from build123d import *

# Parameters (mm, degrees)
Y_KSEKLIK_EKSTR_ZYON1_DEPTH = 2.5
IZIM2_R                     = 1.5
KES_EKSTR_ZYON1_DEPTH       = 11
IZIM3_W                     = 10
IZIM3_H                     = 15
Y_KSEKLIK_EKSTR_ZYON2_DEPTH = 15
IZIM4_W                     = 10
IZIM4_H                     = 10
KES_EKSTR_ZYON2_DEPTH       = 10
IZIM5_R                     = 1.5
KES_EKSTR_ZYON3_DEPTH       = 18


with BuildPart() as part:
    # Çizim1 → Yükseklik-Ekstrüzyon1 (new, symmetric)
    with BuildSketch(Plane.XY):
        with BuildLine():
            Line((22.660097643, 2.30045544), (29.392284146, 8.057892583))
            ThreePointArc((29.392284146, 8.057892583), (30.202384575, 13.188927169), (25.261772713, 14.793337669))
            Line((25.261772713, 14.793337669), (0, 4.329568801))
            Line((0, 4.329568801), (-25.261772713, 14.793337669))
            ThreePointArc((-25.261772713, 14.793337669), (-30.21464291, 13.168805295), (-29.356291498, 8.02747653))
            ThreePointArc((-29.356291498, 8.02747653), (-15.084034375, -6.132217103), (-5, -23.524931034))
            Line((-5, -23.524931034), (-5, -63.524931034))
            Line((-5, -63.524931034), (5, -63.524931034))
            Line((5, -63.524931034), (5, -23.524931034))
            ThreePointArc((5, -23.524931034), (12.493835858, -9.698499239), (22.660097643, 2.30045544))
        make_face()
    extrude(amount=Y_KSEKLIK_EKSTR_ZYON1_DEPTH, both=True)

    # Çizim2 → Kes-Ekstrüzyon1 (cut, symmetric)
    with BuildSketch(Plane.XY.offset(2.5)):
        with Locations((-26.792506443, 11.097819539)):
            Circle(IZIM2_R)
        with Locations((26.792506443, 11.097819539)):
            Circle(IZIM2_R)
    extrude(amount=KES_EKSTR_ZYON1_DEPTH, both=True, mode=Mode.SUBTRACT)

    # Çizim3 → Yükseklik-Ekstrüzyon2 (add)
    with BuildSketch(Plane.XZ.offset(63.524931034)):
        Rectangle(IZIM3_W, IZIM3_H)
    extrude(amount=Y_KSEKLIK_EKSTR_ZYON2_DEPTH)

    # Çizim4 → Kes-Ekstrüzyon2 (cut)
    with BuildSketch(Plane.XZ.offset(78.524931034)):
        Rectangle(IZIM4_W, IZIM4_H)
    extrude(amount=-KES_EKSTR_ZYON2_DEPTH, mode=Mode.SUBTRACT)

    # Çizim5 → Kes-Ekstrüzyon3 (cut)
    with BuildSketch(Plane.XY.offset(7.5)):
        with Locations((0, -73.524931034)):
            Circle(IZIM5_R)
    extrude(amount=-KES_EKSTR_ZYON3_DEPTH, mode=Mode.SUBTRACT)


solid = part.part
Verification items for the finished model (mm, model axes). A direction names the side the tool comes from. Coordinates: 2 decimals unless noted, no trailing zeros. Write each loop counter-clockwise with the first axis right and the second up, starting at its lowest first coordinate (ties: lowest second). Pieces come first, ordered by that corner, then holes. Notation, with made-up numbers: M 26,66.25 L 31,66.25 A29 cw 31,95.25 Z; hole C -35,44.5 d10. An arc over 180 degrees is marked long. Use a Markdown table: item, result.
Q1. Set-up check for faces 1 (the face through (-5, -55, 0)), 2 (the face through (0, -12, -2.5)), 3 (the face through (0, -12, 2.5)), 4 (the face through (12.808, 9.635, 0.035)), 5 (the face through (-1, -75, -5)): record each of +Z, -Z, +X, -X, +Y, -Y from which the full face is reachable in a straight line by a thin tool's end or side.
Reply:
| item | result |
|---|---|
| face 1 | +Z, -Z, -X, -Y |
| face 2 | -Z, +X, -X, +Y |
| face 3 | +Z, +X, -X, +Y |
| face 4 | +Z, -Z, +Y |
| face 5 | +X, -X, -Y |
Q2. Thickness scan on line 1 (Y direction, x = 0, z = -6.2); line 2 (Z direction, x = 1, y = -54.5); line 3 (X direction, y = -58.5, z = 2). Record the ranges inside material, lowest first.
Reply:
| item | result |
|---|---|
| line 1 | y = -78.52 to -75.02, -72.02 to -63.52 |
| line 2 | z = -2.5 to 2.5 |
| line 3 | x = -5 to 5 |
Q3. Go/stop test with flat-tipped pins: P1, Ø5, axis at x = -0.5, y = -72.5, coming from the +Z side; P2, Ø5, axis at x = -3, z = -3.5, coming from the +Y side; P3, Ø8, axis at x = -0.5, z = 0, coming from the -Y side; P4, Ø1.5, axis at x = 0.5, z = 5, coming from the +Y side. Record where each tip stops, or that it passes through.
Reply:
| item | result |
|---|---|
| P1 | stops at z = 7.5 |
| P2 | stops at y = 6.52 |
| P3 | stops at y = -68.52 |
| P4 | stops at y = -63.52 |
Q4. Sectioned sample at B-B, the plane y = 1. Record the boundary of the cut face in (x, z).
Reply:
| item | result |
|---|---|
| outline | M -21.33,-2.5 L 21.34,-2.5 L 21.34,2.5 L -21.33,2.5 Z |
Q5. Sectioned sample at C-C, the plane x = 6.5. Record the boundary of the cut face in (y, z).
Reply:
| item | result |
|---|---|
| outline | M -20.15,-2.5 L 7.02,-2.5 L 7.02,2.5 L -20.15,2.5 Z |
Q6. Draft check along Y on faces 6 (the face through (-28.29, 11.16, 0.04)), 7 (the face through (0, -63.525, -5)), 8 (the face through (0, -71, -7.5)). Enter one of: +Y half, -Y half, draft (parallel to the pull), parting line (faces both ways), or undercut.
Reply:
| item | result |
|---|---|
| face 6 | undercut |
| face 7 | +Y half |
| face 8 | draft |
Q7. Sectioned sample at A-A, the plane z = 1.25. Record the boundary of the cut face in (x, y), plus the area to 3 significant figures.
Reply:
| item | result |
|---|---|
| outline | M -29.36,8.03 A76.39 cw -5,-23.52 L -5,-68.52 L 5,-68.52 L 5,-23.52 A76.39 cw 22.66,2.3 L 29.39,8.06 A4 ccw 25.26,14.79 L 0,4.33 L -25.26,14.79 A4 ccw Z; hole C -26.79,11.1 d3; hole C 26.79,11.1 d3 |
| area | 1,530 mm² |
